```python
from build123d import *

# Parameters (mm, degrees)
SKETCH_W             = 50.292
SKETCH_H             = 10.1092
PAD_DEPTH            = 18.9992
FILLET_R             = 4.064
SKETCH001_W          = 19.05
SKETCH001_H          = 5.08
POCKET_DEPTH         = 10.1102
PAD001_DEPTH         = 2.54
CHAMFER_SIZE         = 1.016
SKETCH003_R          = 0.508
POCKET001_DEPTH      = 25.147
POCKET001_DEPTH_BACK = -25.147


with BuildPart() as part:
    # Sketch → Pad (new body)
    with BuildSketch(Plane.XY):
        Rectangle(SKETCH_W, SKETCH_H)
    extrude(amount=PAD_DEPTH)

    # Fillet
    fillet_edges = [part.edges().sort_by_distance(p)[0] for p in [
        (-25.146, -5.0546, 9.4996),
        (25.146, -5.0546, 9.4996),
        (25.146, 5.0546, 9.4996),
        (-25.146, 5.0546, 9.4996),
    ]]
    fillet(fillet_edges, radius=FILLET_R)

    # Sketch001 (on Face10 of Fillet) → Pocket (cut, through all)
    with BuildSketch(Plane.XZ.offset(5.0546)):
        with Locations((0, 16.4592)):
            Rectangle(SKETCH001_W, SKETCH001_H)
    extrude(amount=-POCKET_DEPTH, mode=Mode.SUBTRACT)

    # Sketch002 → Pad001 (join, symmetric)
    with BuildSketch(Plane.XZ):
        Polygon((9.525, 18.9992), (9.525, 25.3492), (20.523523, 18.9992), align=None)
        Polygon((-9.525, 18.9992), (-9.525, 25.3492), (-20.523523, 18.9992), align=None)
    extrude(amount=PAD001_DEPTH, both=True)

    # Chamfer
    chamfer_edges = [part.edges().sort_by_distance(p)[0] for p in [
        (-15.024261, -2.54, 18.9992),
        (15.024261, -2.54, 18.9992),
        (-15.024261, 2.54, 18.9992),
        (15.024261, 2.54, 18.9992),
    ]]
    chamfer(chamfer_edges, length=CHAMFER_SIZE)

    # Sketch003 → Pocket001 (cut, two sides)
    with BuildSketch(Plane.YZ) as pocket001_sk:
        with Locations((0, 22.6822)):
            Circle(SKETCH003_R)
    extrude(amount=-POCKET001_DEPTH, mode=Mode.SUBTRACT)
    extrude(pocket001_sk.sketch, amount=-POCKET001_DEPTH_BACK, mode=Mode.SUBTRACT)


solid = part.part
```
Read the model definition and answer for the solid it produces. Units are mm, in the model's axes. A direction names the side the tool comes from. Give positions to 0.01 mm unless a question says otherwise; leave off trailing zeros. Order: outer loops, then holes, each group sorted by start corner. A loop starts at its lowest first (then second) coordinate and runs counter-clockwise, first axis right, second up. Notation, with made-up numbers: (-33.75, -31) -> (1.25, -31) arc R20 cw to (1.25, -23) -> close; hole circle Ø3 at (89, 78). An arc over 180 degrees is marked (long way). Write item = value, one per line.
1. A cutting plane is placed at C-C, the plane y = 0. Write down the section's boundary in (x, z) (1 decimal), and give its area (3 significant figures).
Numbers:
outline = (-25.1, 0) -> (25.1, 0) -> (25.1, 19) -> (20.5, 19) -> (15, 22.2) -> (9.5, 22.2) -> (9.5, 13.9) -> (-9.5, 13.9) -> (-9.5, 22.2) -> (-15, 22.2) -> (-20.5, 19) -> (-25.1, 19) -> close; (-13.3, 23.2) -> (-9.5, 23.2) -> (-9.5, 25.3) -> close; (9.5, 23.2) -> (13.3, 23.2) -> (9.5, 25.3) -> close
area = 919 mm²
2. A cutting plane is placed at B-B, the plane x = -11. Write down the section's boundary in (y, z), and give its area (3 significant figures).
Numbers:
outline = (-5.05, 0) -> (5.05, 0) -> (5.05, 19) -> (3.56, 19) -> (2.54, 20.02) -> (2.54, 24.5) -> (-2.54, 24.5) -> (-2.54, 20.02) -> (-3.56, 19) -> (-5.05, 19) -> close; hole circle Ø1.02 at (0, 22.68)
area = 220 mm²
3. Given pin 1 (3 mm diameter, centred on x = 15, y = -2, fed in from +Z); pin 2 (1 mm diameter, centred on y = 4, z = 10, fed in from -X); pin 3 (1.6 mm diameter, centred on x = 14, z = 23.5, fed in from -Y), each flat-ended and moving along its own axis, determine where each tip first touches the part or whether it passes through.
Numbers:
pin_1 = 23.05
pin_2 = -24.28
pin_3 = -2.54
4. A cutting plane is placed at A-A, the plane z = 18.5. Write down the section's boundary in (x, y) (3 decimals), and give its area (3 significant figures).
Numbers:
outline = (-25.146, -0.991) arc R4.064 ccw to (-21.082, -5.055) -> (-9.525, -5.055) -> (-9.525, 5.055) -> (-21.082, 5.055) arc R4.064 ccw to (-25.146, 0.991) -> close; (9.525, -5.055) -> (21.082, -5.055) arc R4.064 ccw to (25.146, -0.991) -> (25.146, 0.991) arc R4.064 ccw to (21.082, 5.055) -> (9.525, 5.055) -> close
area = 302 mm²
5. Straight lines are drawn through the part: line 1 along Z through (x, y) = (-8.5, 0.5); line 2 along Z through (x, y) = (11.55, 0); line 3 along X through (y, z) = (1.5, 15.25) (3 decimals). For each, find the intervals that lie inside material, in ascending order.
Numbers:
line_1 = 0 to 13.92
line_2 = 0 to 22.17, 23.19 to 24.18
line_3 = -25.114 to -9.525, 9.525 to 25.114
6. The mould has two halves that part along Y. Classify faces 4 (the face through (11.693, -0.11, 22.186)), 5 (the face through (9.525, 0, 18)), 6 (the face through (12, 2.54, 22)): +Y half, -Y half, draft (parallel to the pull), parting line (faces both ways), or undercut.
Numbers:
face_4 = undercut
face_5 = draft
face_6 = +Y half
7. For faces 1 (the face through (-15.101, -3.041, 19.514)), 2 (the face through (-9.525, 0, 18)), 3 (the face through (-12, 2.54, 22)), determine the directions among +Z, -Z, +X, -X, +Y, -Y from which every point of the face is accessible in a straight line to the end or side of a thin tool.
Numbers:
face_1 = +Z, +X, -X, -Y
face_2 = +Z, +Y, -Y
face_3 = +Z, +X, -X, +Y
8. A cutting plane is placed at D-D, the plane x = 22. Write down the section's boundary in (y, z), and give its area (3 significant figures).
Numbers:
outline = (-4.95, 0) -> (4.95, 0) -> (4.95, 19) -> (-4.95, 19) -> close
area = 188 mm²
